```python
from build123d import *

# Parameters (mm, degrees)
SKETCH2_W           = 100
SKETCH2_H           = 65
BOSS_EXTRUDE1_DEPTH = 50
SHELL1_T            = 3
SKETCH7_W           = 65
SKETCH7_H           = 3
BOSS_EXTRUDE3_DEPTH = 100
CUT_EXTRUDE1_REACH  = 71.827
SKETCH3_W           = 10
SKETCH3_H           = 65
SKETCH4_R           = 4
SKETCH4_R_2         = 1.6
BOSS_EXTRUDE4_DEPTH = 5


with BuildPart() as part:
    # Sketch2 → Boss-Extrude1 (new body)
    with BuildSketch(Plane(origin=(0, 0, 0), x_dir=(1, 0, 0), z_dir=(0, 1, 0))):
        Rectangle(SKETCH2_W, SKETCH2_H)
    extrude(amount=BOSS_EXTRUDE1_DEPTH)

    # Shell1
    shell1_openings = [part.faces().sort_by_distance(p)[0] for p in [
        (50, 25, 0),
        (0, 50, 0),
    ]]
    offset(amount=SHELL1_T, openings=shell1_openings, kind=Kind.INTERSECTION)

    # Sketch7 → Boss-Extrude3 (add)
    with BuildSketch(Plane(origin=(-50, 0, 0), x_dir=(0, 0, -1), z_dir=(1, 0, 0))):
        with Locations((0, 23.9)):
            Rectangle(SKETCH7_W, SKETCH7_H)
    extrude(amount=BOSS_EXTRUDE3_DEPTH)

    # Sketch3 → Cut-Extrude1 (cut, up to next)
    with BuildSketch(Plane(origin=(0, 25.4, 0), x_dir=(1, 0, 0), z_dir=(0, 1, 0)), mode=Mode.PRIVATE) as cut_extrude1_sk1:
        with Locations((45, 0)):
            Rectangle(SKETCH3_W, SKETCH3_H)
    cut_extrude1_tool1 = extrude(cut_extrude1_sk1.sketch, amount=-CUT_EXTRUDE1_REACH, mode=Mode.PRIVATE) & part.part
    add(cut_extrude1_tool1.solids().sort_by_distance((45, 25.4, 0))[0], mode=Mode.SUBTRACT)

    # Sketch4 → Boss-Extrude4 (add)
    # profile 1 of 4: a face of its own
    with BuildSketch(Plane(origin=(0, 25.4, 0), x_dir=(1, 0, 0), z_dir=(0, 1, 0))):
        with Locations(Location((9.07, 25.5, 0), (0, 0, 90))):
            Circle(SKETCH4_R)
        with Locations(Location((9.07, 25.5, 0), (0, 0, 270))):
            Circle(SKETCH4_R_2, mode=Mode.SUBTRACT)
    # profile 2 of 4: a face of its own
    with BuildSketch(Plane(origin=(0, 25.4, 0), x_dir=(1, 0, 0), z_dir=(0, 1, 0))):
        with Locations(Location((7.8, -22.76, 0), (0, 0, 90))):
            Circle(SKETCH4_R)
        with Locations(Location((7.8, -22.76, 0), (0, 0, 270))):
            Circle(SKETCH4_R_2, mode=Mode.SUBTRACT)
    # profile 3 of 4: a face of its own
    with BuildSketch(Plane(origin=(0, 25.4, 0), x_dir=(1, 0, 0), z_dir=(0, 1, 0))):
        with Locations(Location((-43, -7.52, 0), (0, 0, 90))):
            Circle(SKETCH4_R)
        with Locations(Location((-43, -7.52, 0), (0, 0, 270))):
            Circle(SKETCH4_R_2, mode=Mode.SUBTRACT)
    # profile 4 of 4: a face of its own
    with BuildSketch(Plane(origin=(0, 25.4, 0), x_dir=(1, 0, 0), z_dir=(0, 1, 0))):
        with Locations(Location((-43, 20.42, 0), (0, 0, 90))):
            Circle(SKETCH4_R)
        with Locations(Location((-43, 20.42, 0), (0, 0, 270))):
            Circle(SKETCH4_R_2, mode=Mode.SUBTRACT)
    extrude(amount=BOSS_EXTRUDE4_DEPTH)


solid = part.part
```
Here's how the part is built. I have some questions about the finished solid (model axes, mm). A direction names the side the tool comes from. Give positions to 0.01 mm unless a question says otherwise; leave off trailing zeros. Write each loop counter-clockwise with the first axis right and the second up, starting at its lowest first coordinate (ties: lowest second). Pieces come first, ordered by that corner, then holes. Notation, with made-up numbers: (51, 29.25) -> (61, 29.25) arc R16 ccw to (61, 47.25) -> close; hole circle Ø8 at (25.5, -38.75). An arc over 180 degrees is marked (long way). Use one line per item in the form item = value.
1) Suppose I cut it at A-A (x = 31.5). Please give me the cut outline in (y, z), and give its area (3 significant figures).
Verdict:
outline = (-3, -35.5) -> (50, -35.5) -> (50, -32.5) -> (25.4, -32.5) -> (25.4, 32.5) -> (50, 32.5) -> (50, 35.5) -> (-3, 35.5) -> close; hole (0, -32.5) -> (22.4, -32.5) -> (22.4, 32.5) -> (0, 32.5) -> close
area = 708 mm2
2) Suppose I cut it at C-C (y = 20). Please give me the cut outline in (x, z).
Verdict:
outline = (-53, -35.5) -> (50, -35.5) -> (50, -32.5) -> (-50, -32.5) -> (-50, 32.5) -> (50, 32.5) -> (50, 35.5) -> (-53, 35.5) -> close
3) Suppose I cut it at B-B (z = 22.76). Please give me the cut outline in (x, y).
Verdict:
outline = (-53, -3) -> (50, -3) -> (50, 0) -> (-50, 0) -> (-50, 22.4) -> (40, 22.4) -> (40, 25.4) -> (11.8, 25.4) -> (11.8, 30.4) -> (9.4, 30.4) -> (9.4, 25.4) -> (6.2, 25.4) -> (6.2, 30.4) -> (3.8, 30.4) -> (3.8, 25.4) -> (-50, 25.4) -> (-50, 50) -> (-53, 50) -> close
4) We'd pull the mould along X, two halves only. Please class faces 5 (the face through (-1, 19, 32.5)), 6 (the face through (-43.176, 27.865, -16.424)), 7 (the face through (8.9, 27.9, 21.6)), 8 (the face through (-53, 23, 0)): +X half, -X half, draft (parallel to the pull), parting line (faces both ways), or undercut.
Verdict:
face_5 = draft
face_6 = undercut
face_7 = undercut
face_8 = -X half
5) Suppose I cut it at D-D (x = -43). Please give me the cut outline in (y, z).
Verdict:
outline = (-3, -35.5) -> (50, -35.5) -> (50, -32.5) -> (25.4, -32.5) -> (25.4, -24.42) -> (30.4, -24.42) -> (30.4, -22.02) -> (25.4, -22.02) -> (25.4, -18.82) -> (30.4, -18.82) -> (30.4, -16.42) -> (25.4, -16.42) -> (25.4, 3.52) -> (30.4, 3.52) -> (30.4, 5.92) -> (25.4, 5.92) -> (25.4, 9.12) -> (30.4, 9.12) -> (30.4, 11.52) -> (25.4, 11.52) -> (25.4, 32.5) -> (50, 32.5) -> (50, 35.5) -> (-3, 35.5) -> close; hole (0, -32.5) -> (22.4, -32.5) -> (22.4, 32.5) -> (0, 32.5) -> close
6) I'm going to push flat-ended pins straight in: pin 1 (4 mm diameter, centred on x = 9, z = 23, fed in from +Y); pin 2 (19.5 mm diameter, centred on x = -5.5, z = -13.5, fed in from +Y); pin 3 (5 mm diameter, centred on y = 35, z = 21.5, fed in from +X). Where does each tip first touch, or does it pass through?
Verdict:
pin_1 = 30.4
pin_2 = 25.4
pin_3 = -50
7) If I drill on L1, parallel to X at y = 26.65, z = -20.42; L2, parallel to X at y = 28.45, z = -25.5; L3, parallel to Z at x = 13.5, y = 43, over which ranges is the centre line in solid material (lowest first)? Write a range as [from, to].
Verdict:
L1 = [-53, -50], [-47, -44.6], [-41.4, -39]
L2 = [-53, -50], [5.07, 7.47], [10.67, 13.07]
L3 = [-35.5, -32.5], [32.5, 35.5]
8) On a 3-axis mill with a long thin cutter (end or side, diameter ignored), from which of +Z, -Z, +X, -X, +Y, -Y can I reach the whole of each face in a straight line? I mean faces 1 (the face through (8, 30.4, 21)), 2 (the face through (7.624, 27.865, 26.756)), 3 (the face through (-2, 23, -35.5)), 4 (the face through (-1, 0, 0)). Say none if no direction works.
Verdict:
face_1 = +X, +Y
face_2 = +Y
face_3 = -Z, +X, -X, +Y, -Y
face_4 = +X
